CAD build for the part. Positions are in the model's coordinates, mm. A direction names the side the tool comes from. Round coordinates to 2 decimals unless told otherwise and drop trailing zeros. Order: outer loops, then holes, each group sorted by start corner. A loop starts at its lowest first (then second) coordinate and runs counter-clockwise, first axis right, second up. Notation, with made-up numbers: (22, 80.25) -> (40, 80.25) arc R12 ccw to (40, 101.25) -> close; hole circle Ø2 at (-39.75, 72). An arc over 180 degrees is marked (long way). Return JSON: item names as keys, results as strings. Group by question number.
Q1. Probe line 1 along Y through (x, z) = (19.1, 12.5); line 2 along Y through (x, z) = (21, 17.5); line 3 along X through (y, z) = (72, 19.25). List the from-to ranges inside material, lowest first.
Q2. Cut at B-B (x = 31). Write the cut outline in (y, z), then the cut area to 3 significant figures.
Q3. Cut at A-A (y = 20). Write the cut outline in (x, z), then the cut area to 3 significant figures.
Q4. Which spindle directions (+Z, -Z, +X, -X, +Y, -Y) get a long thin tool onto all of the face, cutting with end or side? Do faces 4 (the flat face through (31.1, 5, 12.3)), 5 (the flat face through (17.5, 44, 13)), 6 (the flat face through (20, 23, 0)). Say none if no direction does.
Q5. Cut at C-C (z = 9.5). Write the cut outline in (x, y), then the cut area to 3 significant figures.
Q6. Cut at D-D (z = 16.75). Write the cut outline in (x, y).
Q7. Flat gauge pins, fed straight in: pin 1 (1 mm diameter, centred on y = 13, z = 16, fed in from +X); pin 2 (14.5 mm diameter, centred on y = 70, z = 12.5, fed in from -X); pin 3 (5 mm diameter, centred on x = 12.5, z = 15, fed in from +Y); pin 4 (2.5 mm diameter, centred on x = 9, z = 10, fed in from -Y). Where does each tip first touch, or does it go through?
Q8. Mould opens along X. For faces 1 (the cylindrical face through (20.035, 81.241, 21.436)), 2 (the flat face through (0, 2, 14)), 3 (the cylindrical face through (29.722, 2.535, 8.334)) say: +X half, -X half, draft (parallel to the pull), parting line (faces both ways), or undercut.
from build123d import *

# Parameters (mm, degrees)
SKETCH1_W           = 40
SKETCH1_H           = 25
BOSS_EXTRUDE1_DEPTH = 5
SKETCH3_W           = 5
SKETCH3_H           = 25
BOSS_EXTRUDE2_DEPTH = 80
SKETCH4_R           = 5.5
CUT_EXTRUDE1_DEPTH  = 92.412526494
SKETCH7_R           = 2.1
CUT_EXTRUDE2_DEPTH  = 93.870878105
FILLET1_R           = 12.5
FILLET2_R           = 2


with BuildPart() as part:
    # Sketch1 → Boss-Extrude1 (new body)
    with BuildSketch(Plane(origin=(0, 0, 0), x_dir=(1, 0, 0), z_dir=(0, 1, 0))):
        with Locations((20, -12.5)):
            Rectangle(SKETCH1_W, SKETCH1_H)
    extrude(amount=BOSS_EXTRUDE1_DEPTH)

    # Sketch3 → Boss-Extrude2 (add)
    with BuildSketch(Plane(origin=(0, 5, 0), x_dir=(1, 0, 0), z_dir=(0, 1, 0))):
        with Locations((20, -12.5)):
            Rectangle(SKETCH3_W, SKETCH3_H)
    extrude(amount=BOSS_EXTRUDE2_DEPTH)

    # Sketch4 → Cut-Extrude1 (cut, through all)
    with BuildSketch(Plane.ZY.offset(-17.5)):
        with Locations((12.5, 70)):
            Circle(SKETCH4_R)
        with Locations((12.5, 20)):
            Circle(SKETCH4_R)
    extrude(amount=-CUT_EXTRUDE1_DEPTH, mode=Mode.SUBTRACT)

    # Sketch7 → Cut-Extrude2 (cut, through all)
    with BuildSketch(Plane(origin=(0, 5, 0), x_dir=(1, 0, 0), z_dir=(0, 1, 0))):
        with Locations(Location((9, -10, 0), (0, 0, 270))):
            Circle(SKETCH7_R)
        with Locations(Location((31, -10, 0), (0, 0, 270))):
            Circle(SKETCH7_R)
    extrude(amount=-CUT_EXTRUDE2_DEPTH, mode=Mode.SUBTRACT)

    # Fillet1
    fillet1_edges = [part.edges().sort_by_distance(p)[0] for p in [
        (20, 85, 0),
        (20, 85, 25),
    ]]
    fillet(fillet1_edges, radius=FILLET1_R - 0.0001)  # a hair under: the kernel refuses the full size

    # Fillet2
    fillet2_edges = [part.edges().sort_by_distance(p)[0] for p in [
        (0, 2.5, 0),
        (40, 2.5, 0),
    ]]
    fillet(fillet2_edges, radius=FILLET2_R)


solid = part.part
Solution:
{
 "1": {"line 1": "y = 0 to 14.5, 25.5 to 64.5, 75.5 to 85", "line 2": "y = 0 to 17.71, 22.29 to 67.71, 72.29 to 83.96", "line 3": "x = 17.5 to 22.5"},
 "2": {"outline": "(0, 0) -> (5, 0) -> (5, 7.9) -> (0, 7.9) -> close; (0, 12.1) -> (5, 12.1) -> (5, 25) -> (0, 25) -> close", "area": "104 mm²"},
 "3": {"outline": "(17.5, 0) -> (22.5, 0) -> (22.5, 7) -> (17.5, 7) -> close; (17.5, 18) -> (22.5, 18) -> (22.5, 25) -> (17.5, 25) -> close", "area": "70.0 mm²"},
 "4": {"face 4": "+Z, -Z, +X, +Y", "face 5": "+Z, -Z, -X, +Y", "face 6": "-Z, +X, -X, +Y, -Y"},
 "5": {"outline": "(0, 0) -> (6.96, 0) -> (6.96, 5) -> (0, 5) -> close; (11.04, 0) -> (28.96, 0) -> (28.96, 5) -> (22.5, 5) -> (22.5, 15.39) -> (17.5, 15.39) -> (17.5, 5) -> (11.04, 5) -> close; (17.5, 24.61) -> (22.5, 24.61) -> (22.5, 65.39) -> (17.5, 65.39) -> close; (17.5, 74.61) -> (22.5, 74.61) -> (22.5, 84.63) -> (17.5, 84.63) -> close; (33.04, 0) -> (40, 0) -> (40, 5) -> (33.04, 5) -> close", "area": "465 mm²"},
 "6": {"outline": "(0, 0) -> (40, 0) -> (40, 5) -> (22.5, 5) -> (22.5, 16.51) -> (17.5, 16.51) -> (17.5, 5) -> (0, 5) -> close; (17.5, 23.49) -> (22.5, 23.49) -> (22.5, 66.51) -> (17.5, 66.51) -> close; (17.5, 73.49) -> (22.5, 73.49) -> (22.5, 84.26) -> (17.5, 84.26) -> close"},
 "7": {"pin 1": "stops at x = 22.5", "pin 2": "stops at x = 17.5", "pin 3": "stops at y = 5", "pin 4": "passes through"},
 "8": {"face 1": "draft", "face 2": "-X half", "face 3": "undercut"}
}
